from build123d import *

# Parameters (mm, degrees)
BOSS_EXTRUDE1_DEPTH      = 609.6
BOSS_EXTRUDE1_DEPTH_BACK = 609.6
SKETCH5_R                = 5.334
CUT_EXTRUDE1_DEPTH       = 16.875
SKETCH6_R                = 5.334
CUT_EXTRUDE2_DEPTH       = 16.875
LPATTERN1_COUNT          = 48
LPATTERN1_PITCH          = 25.4
SKETCH7_W                = 635
SKETCH7_H                = 31.75
CUT_EXTRUDE3_DEPTH       = 70
SKETCH8_R                = 5.334
SKETCH8_W                = 25.4
SKETCH8_H                = 4.1148
CUT_EXTRUDE4_DEPTH       = 70
SKETCH9_R                = 5.334
SKETCH9_W                = 381
SKETCH9_H                = 4.1148
CUT_EXTRUDE5_DEPTH       = 70


with BuildPart() as part:
    # Sketch4 → Boss-Extrude1 (new body, two sides)
    with BuildSketch(Plane(origin=(0, 0, 0), x_dir=(0, 0, -1), z_dir=(1, 0, 0))) as boss_extrude1_sk:
        with BuildLine():
            Line((-15.875, -13.1318), (11.7602, -13.1318))
            ThreePointArc((11.7602, -13.1318), (12.730067661, -12.730067661), (13.1318, -11.7602))
            Line((13.1318, -11.7602), (13.1318, 15.875))
            Line((13.1318, 15.875), (15.875, 15.875))
            Line((15.875, 15.875), (15.875, -11.7602))
            ThreePointArc((15.875, -11.7602), (14.669802983, -14.669802983), (11.7602, -15.875))
            Line((11.7602, -15.875), (-15.875, -15.875))
            Line((-15.875, -15.875), (-15.875, -13.1318))
        make_face()
    extrude(amount=BOSS_EXTRUDE1_DEPTH)
    extrude(boss_extrude1_sk.sketch, amount=-BOSS_EXTRUDE1_DEPTH_BACK)

    # Sketch5 → Cut-Extrude1 (cut, through all)
    with BuildSketch(Plane.XY):
        with Locations((596.9, 0)):
            Circle(SKETCH5_R)
    cut_extrude1 = extrude(amount=-CUT_EXTRUDE1_DEPTH, mode=Mode.SUBTRACT)

    # Sketch6 → Cut-Extrude2 (cut, through all)
    with BuildSketch(Plane(origin=(0, 0, 0), x_dir=(1, 0, 0), z_dir=(0, 1, 0))):
        with Locations((596.9, 0)):
            Circle(SKETCH6_R)
    cut_extrude2 = extrude(amount=-CUT_EXTRUDE2_DEPTH, mode=Mode.SUBTRACT)

    # LPattern1: Cut-Extrude1, Cut-Extrude2 ×48
    with Locations(*[(-i * LPATTERN1_PITCH, 0, 0) for i in range(1, LPATTERN1_COUNT)]):
        add(cut_extrude1, mode=Mode.SUBTRACT)
        add(cut_extrude2, mode=Mode.SUBTRACT)

    # Sketch7 → Cut-Extrude3 (cut)
    with BuildSketch(Plane(origin=(0, 0, -15.875), x_dir=(-1, 0, 0), z_dir=(0, 0, -1))):
        with Locations((-292.1, 0)):
            Rectangle(SKETCH7_W, SKETCH7_H)
    extrude(amount=-CUT_EXTRUDE3_DEPTH, mode=Mode.SUBTRACT)

    # Sketch8 → Cut-Extrude4 (cut)
    with BuildSketch(Plane(origin=(0, 0, -15.875), x_dir=(-1, 0, 0), z_dir=(0, 0, -1))):
        Polygon((50.8, 15.875), (25.4, 15.875), (25.4, -11.7602), (50.8, -11.7602), (50.8, 0), align=None)
        with Locations((38.1, 0)):
            Circle(SKETCH8_R, mode=Mode.SUBTRACT)
        with Locations((38.1, -13.8176)):
            Rectangle(SKETCH8_W, SKETCH8_H)
    extrude(amount=-CUT_EXTRUDE4_DEPTH, mode=Mode.SUBTRACT)

    # Sketch9 → Cut-Extrude5 (cut)
    with BuildSketch(Plane(origin=(0, 0, -15.875), x_dir=(-1, 0, 0), z_dir=(0, 0, -1))):
        Polygon((431.8, 15.875), (50.8, 15.875), (50.8, -11.7602), (431.8, -11.7602), (431.8, 0), align=None)
        with Locations((63.5, 0)):
            Circle(SKETCH9_R, mode=Mode.SUBTRACT)
        with Locations((88.9, 0)):
            Circle(SKETCH9_R, mode=Mode.SUBTRACT)
        with Locations((114.3, 0)):
            Circle(SKETCH9_R, mode=Mode.SUBTRACT)
        with Locations((139.7, 0)):
            Circle(SKETCH9_R, mode=Mode.SUBTRACT)
        with Locations((165.1, 0)):
            Circle(SKETCH9_R, mode=Mode.SUBTRACT)
        with Locations((190.5, 0)):
            Circle(SKETCH9_R, mode=Mode.SUBTRACT)
        with Locations((215.9, 0)):
            Circle(SKETCH9_R, mode=Mode.SUBTRACT)
        with Locations((241.3, 0)):
            Circle(SKETCH9_R, mode=Mode.SUBTRACT)
        with Locations((266.7, 0)):
            Circle(SKETCH9_R, mode=Mode.SUBTRACT)
        with Locations((292.1, 0)):
            Circle(SKETCH9_R, mode=Mode.SUBTRACT)
        with Locations((317.5, 0)):
            Circle(SKETCH9_R, mode=Mode.SUBTRACT)
        with Locations((342.9, 0)):
            Circle(SKETCH9_R, mode=Mode.SUBTRACT)
        with Locations((368.3, 0)):
            Circle(SKETCH9_R, mode=Mode.SUBTRACT)
        with Locations((393.7, 0)):
            Circle(SKETCH9_R, mode=Mode.SUBTRACT)
        with Locations((419.1, 0)):
            Circle(SKETCH9_R, mode=Mode.SUBTRACT)
        with Locations((241.3, -13.8176)):
            Rectangle(SKETCH9_W, SKETCH9_H)
    extrude(amount=-CUT_EXTRUDE5_DEPTH, mode=Mode.SUBTRACT)


solid = part.part
Can you work these out from the model? Positions are in its coordinate system, mm. Coordinates: 2 decimals unless noted, no trailing zeros. Order: outer loops, then holes, each group sorted by start corner. A loop starts at its lowest first (then second) coordinate and runs counter-clockwise, first axis right, second up. Notation, with made-up numbers: M 63.25,47 L 72.25,47 A11 cw 72.25,60 Z; hole C -21,-6.75 d8. An arc over 180 degrees is marked long. Write item = value, one per line.
(1) Suppose I cut it at A-A on x = -495.3. Please give me the cut outline in (y, z) (3 decimals).
Results are:
outline = M -15.875,-11.76 A4.115 ccw -11.76,-15.875 L -5.334,-15.875 L -5.334,-13.132 L -11.76,-13.132 A1.372 cw -13.132,-11.76 L -13.132,-5.334 L -15.875,-5.334 Z; M -15.875,5.334 L -13.132,5.334 L -13.132,15.875 L -15.875,15.875 Z; M 5.334,-15.875 L 15.875,-15.875 L 15.875,-13.132 L 5.334,-13.132 Z
(2) Suppose I cut it at B-B on y = 0. State how many separate pieces and enclosed holes the cut face has, plus the area to 3 significant figures.
Results are:
separate_pieces = 8
enclosed_holes = 0
area = 283 mm2
(3) If we mould it in two halves opening along Z, with no side actions, what happens to faces 1 (the face through (-467.032, 4.498, -14.484)), 2 (the face through (-524.93, -14.48, 3.25)), 3 (the face through (-519.46, -14.64, -14.7)), 4 (the face through (-519, 8, -13.132))? For each: pulls with the +Z half, pulls with the -Z half, needs draft (parallel to the pull), parting line crosses it, or undercut.
Results are:
face_1 = needs draft
face_2 = undercut
face_3 = pulls with the -Z half
face_4 = pulls with the +Z half
(4) Suppose I cut it at D-D on x = -595.5. Please give me the cut outline in (y, z) (3 decimals), plus the area to 3 significant figures.
Results are:
outline = M -15.875,-11.76 A4.115 ccw -11.76,-15.875 L -5.147,-15.875 L -5.147,-13.132 L -11.76,-13.132 A1.372 cw -13.132,-11.76 L -13.132,-5.147 L -15.875,-5.147 Z; M -15.875,5.147 L -13.132,5.147 L -13.132,15.875 L -15.875,15.875 Z; M 5.147,-15.875 L 15.875,-15.875 L 15.875,-13.132 L 5.147,-13.132 Z
area = 107 mm2
(5) For pin 1 Ø4 at (y, z) = (2, -12.5) entering from +X; pin 2 Ø14 at (x, y) = (-546.1, 0) entering from +Z, each with a flat end and sliding along its axis, tell me the tip position at first contact or that it passes through.
Results are:
pin_1 = -431.8
pin_2 = -13.13
(6) Suppose I cut it at C-C on z = 12. Please give me the cut outline in (x, y) (3 decimals), plus the area to 3 significant figures.
Results are:
outline = M -609.6,-15.875 L -431.8,-15.875 L -431.8,-13.132 L -609.6,-13.132 Z
area = 488 mm2
(7) I need wall thicknesses on line 1 along Y through (x, z) = (-443, 11.5) (3 decimals); line 2 along Y through (x, z) = (-596.9, -14) (3 decimals). Which ranges of each line are inside material? Lowest first, please. Write a range as [from, to].
Results are:
line_1 = [-15.875, -13.132]
line_2 = [-15.212, -5.334], [5.334, 15.875]
